CAD build for the part. Positions are in the model's coordinates, mm. A direction names the side the tool comes from. Round coordinates to 2 decimals unless told otherwise and drop trailing zeros. Put each result on its own line as item: value.
```python
from build123d import *

# Parameters (mm, degrees)
SKETCH1_R               = 9.926666649
BOSS_EXTRUDE1_DEPTH     = 2.54
SKETCH2_R               = 12.466666649
BOSS_EXTRUDE2_DEPTH     = 1.27
FILLET1_R               = 0.635
CUT_EXTRUDE1_DEPTH      = 20.718919442
CUT_EXTRUDE1_DEPTH_BACK = 20.718919442
SKETCH4_W               = 27.24769987
SKETCH4_H               = 6.35
FILLET2_R               = 6.35


with BuildPart() as part:
    # Sketch1 → Boss-Extrude1 (new body)
    with BuildSketch(Plane(origin=(0, 0, 0), x_dir=(1, 0, 0), z_dir=(0, 1, 0))):
        with Locations(Location((0, 0, 0), (0, 0, 270))):
            Circle(SKETCH1_R)
    extrude(amount=BOSS_EXTRUDE1_DEPTH)

    # Sketch2 → Boss-Extrude2 (add)
    with BuildSketch(Plane(origin=(0, 2.54, 0), x_dir=(1, 0, 0), z_dir=(0, 1, 0))):
        with Locations(Location((0, 0, 0), (0, 0, 270))):
            Circle(SKETCH2_R)
    extrude(amount=BOSS_EXTRUDE2_DEPTH)

    # Sketch3 → Revolve1 (revolve)
    with BuildSketch(Plane.XY):
        with BuildLine():
            Line((0, 8.831773608), (0, 3.81))
            Line((0, 3.81), (-11.196666649, 3.81))
            ThreePointArc((-11.196666649, 3.81), (-6.127083682, 7.49980126), (0, 8.831773608))
        make_face()
    revolve(axis=Axis((0, 8.831773608, 0), (0, -1, 0)))

    # Fillet1
    fillet1_edges = [part.edges().sort_by_distance(p)[0] for p in [
        (0, 3.81, -12.466666649),
    ]]
    fillet(fillet1_edges, radius=FILLET1_R)

    # Sketch4 → Cut-Extrude1 (cut, two sides: drawn at the far end of the back side and taken through both)
    with BuildSketch(Plane.XY.offset(-CUT_EXTRUDE1_DEPTH_BACK)):
        with Locations((-1.310749411, 9.525)):
            Rectangle(SKETCH4_W, SKETCH4_H)
    extrude(amount=CUT_EXTRUDE1_DEPTH + CUT_EXTRUDE1_DEPTH_BACK, mode=Mode.SUBTRACT)

    # Fillet2
    fillet2_edges = [part.edges().sort_by_distance(p)[0] for p in [
        (8.22955279, 6.35, -5e-09),
    ]]
    fillet(fillet2_edges, radius=FILLET2_R)


solid = part.part
```
Item 1: Tool access for faces 1 (the flat face through (-9, 3.81, -7)), 2 (the cylindrical face through (10.512, 2.853, 6.702)), 3 (the flat face through (-10.1, 2.54, -1)): list every direction of +Z, -Z, +X, -X, +Y, -Y with a clear straight run to the whole face (end or side of a thin tool).
Answers below:
face 1: +Y
face 2: +Y, -Y
face 3: -Y
Item 2: Pin check, flat tips, straight feed: P1, Ø2, axis at x = -4, y = 1.5, coming from the -Z side; P2, Ø1, axis at x = -5.5, z = -10, coming from the +Y side; P3, Ø1, axis at x = -9, z = -8.5, coming from the +Y side. Stop position of each tip, or through.
Answers below:
P1: z = -9.46
P2: y = 4.12
P3: y = 3.81
Item 3: Probe line 1 along Y through (x, z) = (-10.5, -5.5); line 2 along X through (y, z) = (4.25, -4.25); line 3 along Y through (x, z) = (7, 3.75). List the from-to ranges inside material, lowest first. Write a range as [from, to].
Answers below:
line 1: [2.54, 3.81]
line 2: [-9.91, 9.91]
line 3: [0, 6.06]
